For this review, take the finished solid that the model builds, in its own axes (mm). A direction names the side the tool comes from. Coordinates: 2 decimals unless noted, no trailing zeros. Loops run counter-clockwise (first coordinate to the right, second up) from the corner with the lowest first, then second, coordinate; pieces in that order, holes last. Notation, with made-up numbers: M 2,13 L 15,13 A19 ccw 15,47 Z; hole C 66.25,61 d3. An arc over 180 degrees is marked long. Put each result on its own line as item: value.
```python
from build123d import *

# Parameters (mm, degrees)
BOSS_EXTRUDE1_DEPTH     = 222.25
CUT_EXTRUDE1_DEPTH      = 1
CUT_EXTRUDE1_DEPTH_BACK = 445.5


with BuildPart() as part:
    # Sketch1 → Boss-Extrude1 (new body, symmetric)
    with BuildSketch(Plane.XY):
        with BuildLine():
            Line((0, 44.45), (1066.8, 44.45))
            ThreePointArc((1066.8, 44.45), (1111.25, 0), (1066.8, -44.45))
            Line((1066.8, -44.45), (0, -44.45))
            ThreePointArc((0, -44.45), (-44.45, 0), (0, 44.45))
        make_face()
    extrude(amount=BOSS_EXTRUDE1_DEPTH, both=True)

    # Sketch2 → Cut-Extrude1 (cut, two sides)
    with BuildSketch(Plane(origin=(0, 0, -222.25), x_dir=(-1, 0, 0), z_dir=(0, 0, -1))) as cut_extrude1_sk:
        with BuildLine():
            Line((-1066.8, 38.1), (0, 38.1))
            ThreePointArc((0, 38.1), (38.1, 0), (0, -38.1))
            Line((0, -38.1), (-1066.8, -38.1))
            ThreePointArc((-1066.8, -38.1), (-1104.9, 0), (-1066.8, 38.1))
        make_face()
    extrude(amount=CUT_EXTRUDE1_DEPTH, mode=Mode.SUBTRACT)
    extrude(cut_extrude1_sk.sketch, amount=-CUT_EXTRUDE1_DEPTH_BACK, mode=Mode.SUBTRACT)


solid = part.part
```
(1) Add section A-A (z = 34). Write out the cut boundary in (x, y), plus the area to 3 significant figures.
Determined:
outline: M 0,-44.45 L 1066.8,-44.45 A44.45 ccw 1066.8,44.45 L 0,44.45 A44.45 ccw Z; hole M 0,-38.1 L 1066.8,-38.1 A38.1 ccw 1066.8,38.1 L 0,38.1 A38.1 ccw Z
area: 15,200 mm^2
(2) Wall thickness on line 1 along Y through (x, z) = (325, -139.5); line 2 along X through (y, z) = (7, 103.5); line 3 along X through (y, z) = (22, 159): over which ranges is each line inside the solid? List them lowest first. Write a range as [from, to].
Determined:
line 1: y = [-44.45, -38.1], [38.1, 44.45]
line 2: x = [-43.9, -37.45], [1104.25, 1110.7]
line 3: x = [-38.62, -31.11], [1097.91, 1105.42]
(3) Add section C-C (y = 0). Write out the cut boundary in (x, z), plus the area to 3 significant figures.
Determined:
outline: M -44.45,-222.25 L -38.1,-222.25 L -38.1,222.25 L -44.45,222.25 Z; M 1104.9,-222.25 L 1111.25,-222.25 L 1111.25,222.25 L 1104.9,222.25 Z
area: 5,650 mm^2
(4) Add section B-B (x = 675). Write out the cut boundary in (y, z).
Determined:
outline: M -44.45,-222.25 L -38.1,-222.25 L -38.1,222.25 L -44.45,222.25 Z; M 38.1,-222.25 L 44.45,-222.25 L 44.45,222.25 L 38.1,222.25 Z
(5) Tool access review of faces 1 (the cylindrical face through (1104.89, -0.84, -3.11)), 2 (the flat face through (541, -44.45, 3)): name each direction out of +Z, -Z, +X, -X, +Y, -Y from which nothing blocks a thin tool from reaching the whole face with its end or side.
Determined:
face 1: +Z, -Z
face 2: +Z, -Z, +X, -X, -Y
(6) For pin 1 (6 mm diameter, centred on y = 17.5, z = 51, fed in from -X); pin 2 (5 mm diameter, centred on y = -30.5, z = -167, fed in from +X), all flat-tipped, find the tip position at first contact; note any pin that passes through.
Determined:
pin 1: stops at x = -42.02
pin 2: stops at x = 1101.32
(7) Draft analysis for pull direction Y (two halves, no side actions). For faces 3 (the cylindrical face through (1111.24, 0.98, 3.11)), 4 (the flat face through (526, -38.1, -3)), 5 (the flat face through (536, 40, 222.25)), state which applies: +Y half, -Y half, draft (parallel to the pull), parting line (faces both ways), or undercut.
Determined:
face 3: parting line
face 4: undercut
face 5: draft
